from build123d import *

# Parameters (mm, degrees)
SKETCH1_R           = 47.85
BOSS_EXTRUDE1_DEPTH = 3
SKETCH2_R           = 7.5
CUT_EXTRUDE1_DEPTH  = 6
FILLET2_R           = 4


with BuildPart() as part:
    # Sketch1 → Boss-Extrude1 (new body)
    with BuildSketch(Plane.XY):
        Circle(SKETCH1_R)
    extrude(amount=BOSS_EXTRUDE1_DEPTH)

    # Sketch2 → Cut-Extrude1 (cut)
    with BuildSketch(Plane.XY.offset(3)):
        Circle(SKETCH2_R)
    extrude(amount=-CUT_EXTRUDE1_DEPTH, mode=Mode.SUBTRACT)

    # Fillet2
    # the kernel refuses this fillet: 4 mm, written as the material it takes off along each edge
    with BuildSketch(Plane(origin=(0, 0, 3), x_dir=(1, 0, 0), z_dir=(0, -1, 0))) as fillet2_piece_1:
        with BuildLine():
            CenterArc((43.977016654, -4), FILLET2_R, 14.477512186, 75.522487814)
            Line((43.977016654, 0), (43.977016654, 0.08))
            Line((43.977016654, 0.08), (47.85, 0.08))
            Line((47.85, 0.08), (47.93, 0))
            ThreePointArc((47.93, 0), (47.93, -1.5), (47.927459667, -2.98))
            Line((47.927459667, -2.98), (47.85, -3))
        make_face()
    revolve(axis=Axis((0, 0, 3), (0, 0, 1)), mode=Mode.SUBTRACT)


solid = part.part
Source: CAD feature listing. Evaluate the final solid. Frame: model axes, mm. Round coordinates to 2 decimals unless told otherwise and drop trailing zeros. Write each loop counter-clockwise with the first axis right and the second up, starting at its lowest first coordinate (ties: lowest second). Pieces come first, ordered by that corner, then holes. Notation, with made-up numbers: M -39.5,-18 L -20.5,-18 A15 ccw -20.5,-10 Z; hole C -33.75,88.25 d10. An arc over 180 degrees is marked long. One line per item, written item: value. Start each with the question number.
Item 1: Pin query (flat end, axial travel): pin 1 (1 mm diameter, centred on x = 21.5, z = 0.5, fed in from +Y); pin 2 (1 mm diameter, centred on x = 10.5, z = 1, fed in from -Y). Return the tip coordinate at first contact, or that it passes through.
Item 2: Section query C-C (z = 2.05). Return the cut outline in (x, y), plus the area to 3 significant figures.
Item 3: Ray query, L1, parallel to Y at x = 0, z = 2.25; L2, parallel to Y at x = 0, z = 1.4; L3, parallel to X at y = -23.5, z = 2.25. Return the intervals inside material, ascending. Write a range as from..to.
Item 4: Mould query, pull axis X, two halves, no side actions, for faces 1 (the flat face through (-1, -9, 3)), 2 (the cylindrical face through (-7.493, 0.33, 1.521)). Classes: pulls with the +X half, pulls with the -X half, needs draft (parallel to the pull), parting line crosses it, or undercut.
Item 5: Section query A-A (y = 0). Return the cut outline in (x, z).
Result set:
1. pin 1: stops at y = 42.88
1. pin 2: stops at y = -46.54
2. outline: C 0,0 d93.13; hole C 0,0 d15
2. area: 6,640 mm²
3. L1: y = -46.31..-7.5, 7.5..46.31
3. L2: y = -47.18..-7.5, 7.5..47.18
3. L3: x = -39.9..39.9
4. face 1: needs draft
4. face 2: undercut
5. outline: M -47.85,0 L -7.5,0 L -7.5,3 L -43.98,3 A4 ccw Z; M 7.5,0 L 47.85,0 A4 ccw 43.98,3 L 7.5,3 Z
